from build123d import *

# Parameters (mm, degrees)
BOSS_EXTRUDE1_DEPTH   = 10
BOSS_EXTRUDE1_2_DEPTH = 10
BOSS_EXTRUDE1_3_DEPTH = 10
BOSS_EXTRUDE1_4_DEPTH = 10
BOSS_EXTRUDE2_DEPTH   = 2


with BuildPart() as part:
    # Sketch1 → Boss-Extrude1 (new body)
    with BuildSketch(Plane.XY):
        Polygon((-45.029672623, -17.414149003), (-45.029672623, -12.296865077), (31.479998469, 9.563040949), (31.479998469, -17.414149003), align=None)
        Polygon((28.479998469, -14.414149003), (-41.520001531, -14.414149003), (28.479998469, 5.585850997), align=None, mode=Mode.SUBTRACT)
    extrude(amount=BOSS_EXTRUDE1_DEPTH)



with BuildPart() as body_2:
    # Sketch1 → Boss-Extrude1 2 (new body)
    with BuildSketch(Plane.XY):
        Polygon((-20.099836697, -11.414149003), (-10.005608589, -8.530083829), (-10.005608589, -11.414149003), align=None)
    extrude(amount=BOSS_EXTRUDE1_2_DEPTH)


with BuildPart() as body_3:
    # Sketch1 → Boss-Extrude1 3 (new body)
    with BuildSketch(Plane.XY):
        Polygon((-7.005608589, -7.672940972), (8.872659236, -3.136293022), (8.872659236, -11.414149003), (-7.005608589, -11.414149003), align=None)
    extrude(amount=BOSS_EXTRUDE1_3_DEPTH)


with BuildPart() as body_4:
    # Sketch1 → Boss-Extrude1 4 (new body)
    with BuildSketch(Plane.XY):
        Polygon((11.872659236, -2.279150165), (25.479998469, 1.608661044), (25.479998469, -11.414149003), (11.872659236, -11.414149003), align=None)
    extrude(amount=BOSS_EXTRUDE1_4_DEPTH)


with BuildPart() as part_1:
    add(part.part)

    add(body_2.part)  # Boss-Extrude2 merges body 2

    add(body_3.part)  # Boss-Extrude2 merges body 3

    add(body_4.part)  # Boss-Extrude2 merges body 4
    # Sketch2 → Boss-Extrude2 (add)
    with BuildSketch(Plane(origin=(0, 0, 0), x_dir=(-1, 0, 0), z_dir=(0, 0, -1))):
        Polygon((-31.479998469, 9.563040949), (45.029672623, -12.296865077), (45.029672623, -17.414149003), (-31.479998469, -17.414149003), align=None)
    extrude(amount=BOSS_EXTRUDE2_DEPTH)


solid = part_1.part
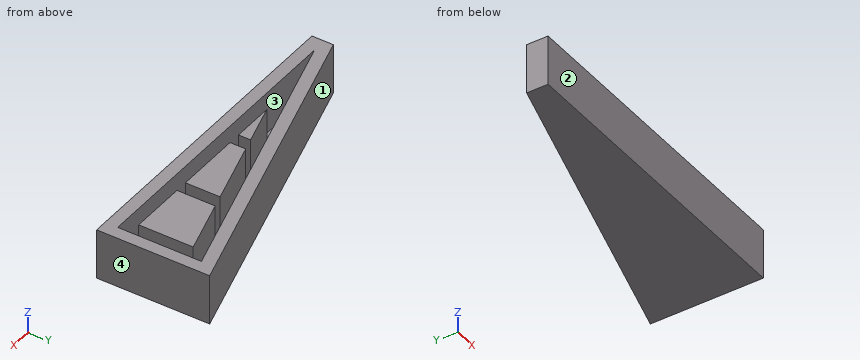
Can you work these out from the model? Positions are in its coordinate system, mm. Face numbers are marked on the shaded views. Give positions to 0.01 mm unless a question says otherwise; leave off trailing zeros. Loops run counter-clockwise (first coordinate to the right, second up) from the corner with the lowest first, then second, coordinate; pieces in that order, holes last. Notation, with made-up numbers: M 15,26.25 L 42,26.25 A13 ccw 42,49.25 Z; hole C 62.5,31.5 d9. An arc over 180 degrees is marked long. One line per item, written item: value. Start each with the question number.
1) If we section it at C-C, the plane y = -4.5: Write out the boundary of the cut face in (x, z).
2) I'm going to push flat-ended pins straight in: pin 1 (1.5 mm diameter, centred on x = -33.5, z = 5.5, fed in from +Y); pin 2 (5 mm diameter, centred on x = -31, z = 8.5, fed in from +Y); pin 3 (3 mm diameter, centred on x = 6, z = 6.5, fed in from +Y). Where does each tip first touch, or does it pass through?
3) If we section it at A-A, the plane z = 6: Write out the boundary of the cut face in (x, y), and give its area (4 significant figures).
4) If we section it at B-B, the plane x = 6.5: Write out the boundary of the cut face in (y, z).
5) Thinking about a two-plate mould opening in Y: for the marked faces 1, 2, 3 and 4, which applies, +Y half, -Y half, draft (parallel to the pull), parting line (faces both ways), or undercut?
6) If we section it at D-D, the plane x = -25: Write out the boundary of the cut face in (y, z), and give its area (3 significant figures).
7) If I drill on line 1 (Y direction, x = -4.5, z = 2.75); line 2 (Z direction, x = -10.5, y = -13.5); line 3 (Y direction, x = -6, z = 8.75), over which ranges is the centre line in solid material (lowest first)? Write a range as [from, to].
Completed:
1. outline: M -17.74,-2 L 31.48,-2 L 31.48,10 L 28.48,10 L 28.48,0 L 25.48,0 L 25.48,10 L 11.87,10 L 11.87,0 L 8.87,0 L 8.87,10 L 4.1,10 L 4.1,0 L -6.82,0 L -6.82,10 L -17.74,10 Z
2. pin 1: stops at y = -8.79
2. pin 2: stops at y = -7.57
2. pin 3: stops at y = 2.71
3. outline: M -45.03,-17.41 L 31.48,-17.41 L 31.48,9.56 L -45.03,-12.3 Z; M -20.1,-11.41 L -10.01,-11.41 L -10.01,-8.53 Z; M -7.01,-11.41 L 8.87,-11.41 L 8.87,-3.14 L -7.01,-7.67 Z; M 11.87,-11.41 L 25.48,-11.41 L 25.48,1.61 L 11.87,-2.28 Z; hole M -41.52,-14.41 L 28.48,-14.41 L 28.48,5.59 Z
3. area: 788.5 mm^2
4. outline: M -17.41,-2 L 2.43,-2 L 2.43,10 L -0.69,10 L -0.69,0 L -3.81,0 L -3.81,10 L -11.41,10 L -11.41,0 L -14.41,0 L -14.41,10 L -17.41,10 Z
5. face 1: +Y half
5. face 2: -Y half
5. face 3: undercut
5. face 4: draft
6. outline: M -17.41,-2 L -6.57,-2 L -6.57,10 L -9.69,10 L -9.69,0 L -14.41,0 L -14.41,10 L -17.41,10 Z
6. area: 82.9 mm^2
7. line 1: y = [-17.41, -14.41], [-11.41, -6.96], [-3.84, -0.72]
7. line 2: z = [-2, 0]
7. line 3: y = [-17.41, -14.41], [-11.41, -7.39], [-4.27, -1.15]
